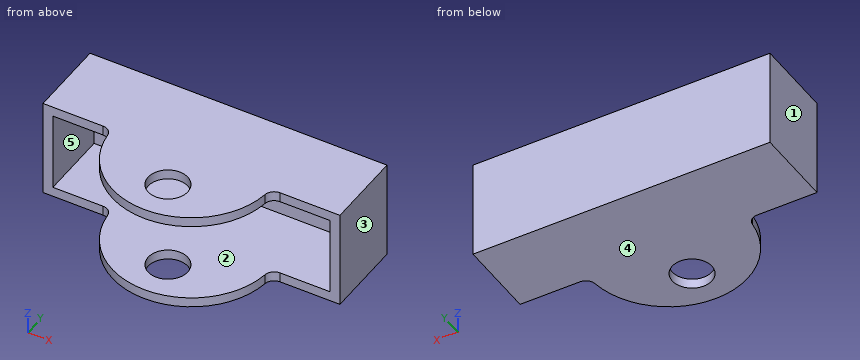
```python
from build123d import *

# Parameters (mm, degrees)
SKETCH1_W               = 150
SKETCH1_H               = 40
SKETCH1_R               = 10
BOSS_EXTRUDE1_DEPTH     = 50
SHELL2_T                = -5
FILLET1_R               = 5
CUT_EXTRUDE2_DEPTH      = 121.519707932
CUT_EXTRUDE2_DEPTH_BACK = 121.519707932
SKETCH1_4_R             = 10


with BuildPart() as part:
    # Sketch1 → Boss-Extrude1 (new body)
    # profile 1 of 3: a face of its own
    with BuildSketch(Plane.XY):
        with Locations((0, -20)):
            Rectangle(SKETCH1_W, SKETCH1_H)
    # profile 2 of 3: a face of its own
    with BuildSketch(Plane.XY):
        with BuildLine():
            Line((40, -40), (-40, -40))
            ThreePointArc((-40, -40), (0, -80), (40, -40))
        make_face()
        with Locations((0, -60)):
            Circle(SKETCH1_R, mode=Mode.SUBTRACT)
    # profile 3 of 3: a face of its own
    with BuildSketch(Plane.XY):
        with Locations((0, -60)):
            Circle(SKETCH1_R)
    extrude(amount=BOSS_EXTRUDE1_DEPTH)

    # Shell2
    shell2_openings = [part.faces().sort_by_distance(p)[0] for p in [
        (57.5, -40, 25),
        (0, -80, 25),
        (-57.5, -40, 25),
    ]]
    offset(amount=SHELL2_T, openings=shell2_openings, kind=Kind.INTERSECTION)

    # Fillet1
    fillet1_edges = [part.edges().sort_by_distance(p)[0] for p in [
        (40, -40, 47.5),
        (-40, -40, 47.5),
        (40, -40, 2.5),
        (-40, -40, 2.5),
    ]]
    fillet(fillet1_edges, radius=FILLET1_R)

    # Sketch1_4 → Cut-Extrude2 (cut, two sides: drawn at the far end of the back side and taken through both)
    with BuildSketch(Plane.XY.offset(-CUT_EXTRUDE2_DEPTH_BACK)):
        with Locations((0, -60)):
            Circle(SKETCH1_4_R)
    extrude(amount=CUT_EXTRUDE2_DEPTH + CUT_EXTRUDE2_DEPTH_BACK, mode=Mode.SUBTRACT)


solid = part.part
```
Design review of the part built by this model. Coordinates are the model's own, in mm. Face numbers are marked on the shaded views. A direction names the side the tool comes from. Round coordinates to 2 decimals unless told otherwise and drop trailing zeros. Write each loop counter-clockwise with the first axis right and the second up, starting at its lowest first coordinate (ties: lowest second). Pieces come first, ordered by that corner, then holes.
Item 1: We need section B-B on y = -21. Write out the cut boundary in (x, z), and give its area (3 significant figures).
Item 2: For probe 1 along Z at (x, y) = (44.5, -38); probe 2 along Y at (x, z) = (0, 2.7); probe 3 along X at (y, z) = (-7, 21), list the stretches that pass through material, from the lowest coordinate up.
Item 3: We need section D-D on z = 19. Write out the cut boundary in (x, y), and give its area (3 significant figures).
Item 4: For the marked faces 1 and 2, list the 3-axis set-ups (+Z, -Z, +X, -X, +Y, -Y) from which the entire face can be reached by the end or side of a thin tool; tool diameter is ignored.
Item 5: Clearance check with flat-ended pins moving along their axes: pin 1 Ø12 at (x, z) = (15.5, 17.5) entering from -Y; pin 2 Ø24 at (x, z) = (-59, 14.5) entering from -Y. State where each tip first meets the part, or that it passes through.
Item 6: We need section A-A on x = 0. Write out the cut boundary in (y, z), and give its area (3 significant figures).
Item 7: The part is to be moulded in two halves that separate along X. For the marked faces 3, 4 and 5, say which applies: +X half, -X half, draft (parallel to the pull), parting line (faces both ways), or undercut.
Item 8: We need section C-C on y = -54. Write out the cut boundary in (x, z), and give its area (3 significant figures).
Returned:
1. outline: (-75, 0) - (75, 0) - (75, 50) - (-75, 50) - close; hole (-70, 5) - (70, 5) - (70, 45) - (-70, 45) - close
1. area: 1,900 mm2
2. probe 1: z = 0 to 5, 45 to 50
2. probe 2: y = -80 to -70, -50 to 0
2. probe 3: x = -75 to -70, 70 to 75
3. outline: (-75, -40) - (-70, -40) - (-70, -5) - (70, -5) - (70, -40) - (75, -40) - (75, 0) - (-75, 0) - close
3. area: 1,100 mm2
4. face 1: +Z, -Z, -X, +Y, -Y
4. face 2: -Y
5. pin 1: stops at y = -5
5. pin 2: stops at y = -40
6. outline: (-80, 0) - (-70, 0) - (-70, 5) - (-80, 5) - close; (-80, 45) - (-70, 45) - (-70, 50) - (-80, 50) - close; (-50, 0) - (0, 0) - (0, 50) - (-50, 50) - (-50, 45) - (-5, 45) - (-5, 5) - (-50, 5) - close
6. area: 800 mm2
7. face 3: +X half
7. face 4: draft
7. face 5: undercut
8. outline: (-37.47, 0) - (-8, 0) - (-8, 5) - (-37.47, 5) - close; (-37.47, 45) - (-8, 45) - (-8, 50) - (-37.47, 50) - close; (8, 0) - (37.47, 0) - (37.47, 5) - (8, 5) - close; (8, 45) - (37.47, 45) - (37.47, 50) - (8, 50) - close
8. area: 589 mm2
